```python
from build123d import *

# Parameters (mm, degrees)
SKETCH_1_R          = 2.84
EXTRUDE_1_DEPTH     = 3
SKETCH_2_R          = 1.5
EXTRUDE_2_DEPTH     = 30
CUT_EXTRUDE_1_DEPTH = 2


with BuildPart() as part:
    # 草图1 → 凸台-拉伸1 (new body)
    with BuildSketch(Plane.XY):
        Circle(SKETCH_1_R)
    extrude(amount=EXTRUDE_1_DEPTH)

    # 草图2 → 凸台-拉伸2 (add)
    with BuildSketch(Plane(origin=(0, 0, 0), x_dir=(-1, 0, 0), z_dir=(0, 0, -1))):
        with Locations(Location((0, 0, 0), (0, 0, 180))):
            Circle(SKETCH_2_R)
    extrude(amount=EXTRUDE_2_DEPTH)

    # 草图3 → 切除-拉伸1 (cut)
    with BuildSketch(Plane.XY.offset(3)):
        Polygon((0.912581429, 1.526213769), (-0.865449181, 1.553425585), (-1.77803061, 0.027211816), (-0.912581429, -1.526213769), (0.865449181, -1.553425585), (1.77803061, -0.027211816), align=None)
    extrude(amount=-CUT_EXTRUDE_1_DEPTH, mode=Mode.SUBTRACT)


solid = part.part
```
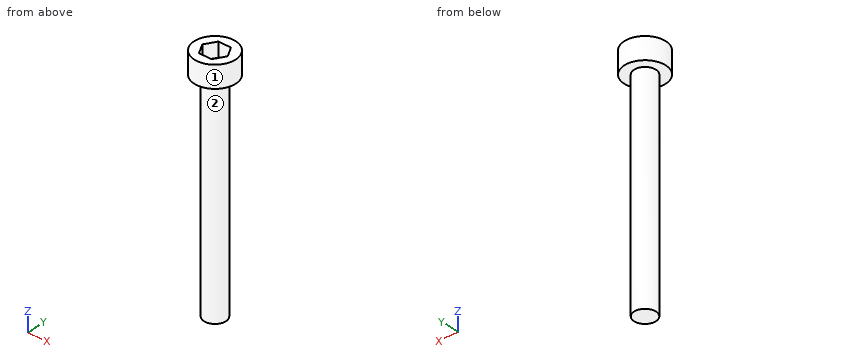
Build history of the part. All positions in model axes, mm. Face numbers are marked on the shaded views. A direction names the side the tool comes from. Give positions to 0.01 mm unless a question says otherwise; leave off trailing zeros. Loops run counter-clockwise (first coordinate to the right, second up) from the corner with the lowest first, then second, coordinate; pieces in that order, holes last. Notation, with made-up numbers: (-30, -32.75) - (29, -32.75) arc R21 cw to (29, -3.75) - close; hole circle Ø9 at (11, 79.5). An arc over 180 degrees is marked (long way). Use a Markdown table: item, result.
(1) Which spindle directions (+Z, -Z, +X, -X, +Y, -Y) get a long thin tool onto all of the face, cutting with end or side? Do the marked faces 1 and 2. Say none if no direction does.
Taken from the geometry:
| item | result |
|---|---|
| face 1 | +Z, -Z |
| face 2 | -Z |
(2) Drop flat-ended pins along their axis: pin 1 Ø1.5 at (y, z) = (1.5, -17.5) entering from +X; pin 2 Ø3 at (x, z) = (-1, -11) entering from +Y; pin 3 Ø2.5 at (x, y) = (-0.5, -0.5) entering from +Z; pin 4 Ø3 at (y, z) = (0.5, -6) entering from -X. Give the stop position or say it passes through.
Taken from the geometry:
| item | result |
|---|---|
| pin 1 | x = 1.3 |
| pin 2 | y = 1.5 |
| pin 3 | z = 3 |
| pin 4 | x = -1.5 |
(3) Band-saw the part on B-B (z = -23). Give the cut face in (x, y).
Taken from the geometry:
| item | result |
|---|---|
| outline | circle Ø3 at (0, 0) |
(4) Band-saw the part on D-D (x = -2.35). Give the cut face in (y, z).
Taken from the geometry:
| item | result |
|---|---|
| outline | (-1.59, 0) - (1.59, 0) - (1.59, 3) - (-1.59, 3) - close |
(5) Wall check: line 1 along Z through (x, y) = (0.9, 2); line 2 along Z through (x, y) = (1, 0.55); line 3 along X through (y, z) = (0.1, -7). Give the ranges that are in metal, low to high.
Taken from the geometry:
| item | result |
|---|---|
| line 1 | 0 to 3 |
| line 2 | -30 to 1 |
| line 3 | -1.5 to 1.5 |
(6) Band-saw the part on A-A (x = -0.25). Give the cut face in (y, z).
Taken from the geometry:
| item | result |
|---|---|
| outline | (-2.83, 0) - (-1.48, 0) - (-1.48, -30) - (1.48, -30) - (1.48, 0) - (2.83, 0) - (2.83, 3) - (1.54, 3) - (1.54, 1) - (-1.54, 1) - (-1.54, 3) - (-2.83, 3) - close |
(7) Band-saw the part on C-C (y = 0.95). Give the cut face in (x, z).
Taken from the geometry:
| item | result |
|---|---|
| outline | (-2.68, 0) - (-1.16, 0) - (-1.16, -30) - (1.16, -30) - (1.16, 0) - (2.68, 0) - (2.68, 3) - (1.23, 3) - (1.23, 1) - (-1.23, 1) - (-1.23, 3) - (-2.68, 3) - close |
